Answer from the drawing. Dimensions are ordinates in mm from the lowest x, y and z of the part. A direction names the side the tool comes from. Give positions to 0.01 mm unless a question says otherwise; leave off trailing zeros. Write each loop counter-clockwise with the first axis right and the second up, starting at its lowest first coordinate (ties: lowest second). Pieces come first, ordered by that corner, then holes. Notation, with made-up numbers: (84, 60) -> (108, 60) arc R4 cw to (108, 67) -> close; hole circle Ø10 at (44.5, 56.5). An arc over 180 degrees is marked (long way). Write item = value, one per line.
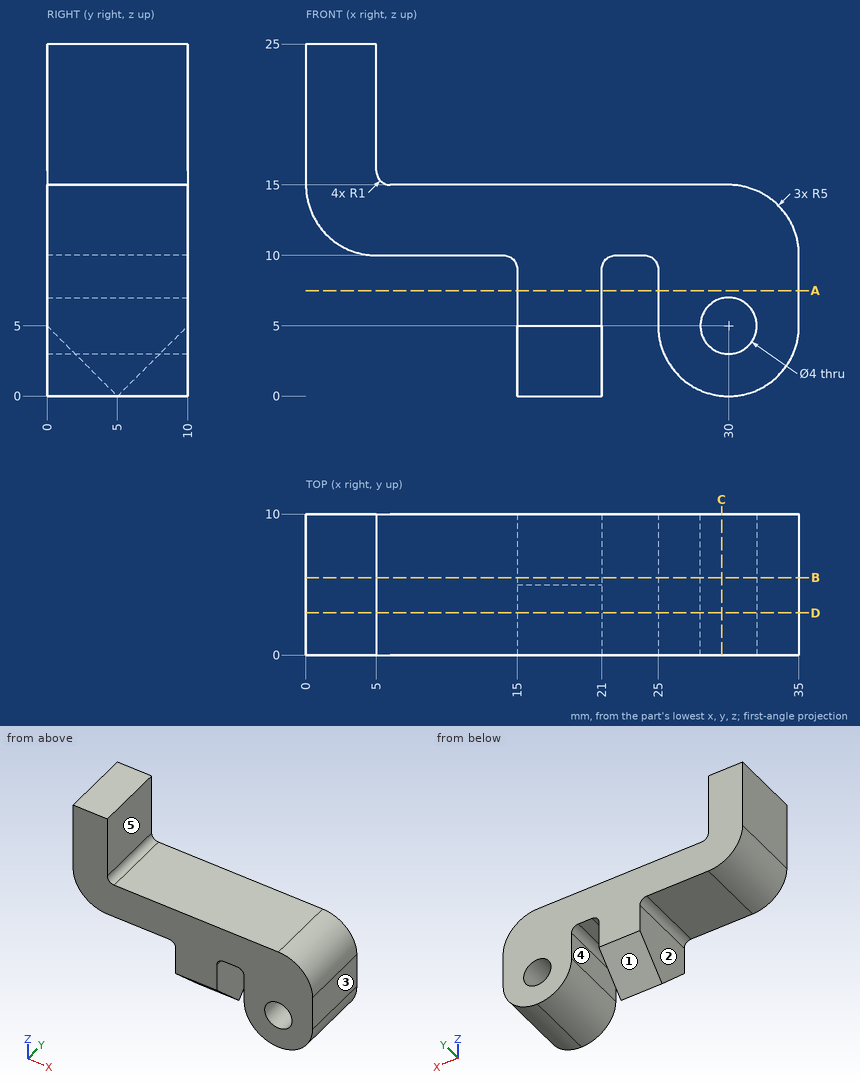
(1) The part is cut by section A-A on z = 7.5. Determine the outline of the cut face in (x, y).
Checks:
outline = (15, 0) -> (21, 0) -> (21, 10) -> (15, 10) -> close; (25, 0) -> (35, 0) -> (35, 10) -> (25, 10) -> close
(2) Consider L1, parallel to Z at x = 9, y = 6.75; L2, parallel to X at y = 8, z = 7.25; L3, parallel to X at y = 1, z = 5.75. Determine where each line is inside the solid, lowest interval first.
Checks:
L1 = 10 to 15
L2 = 15 to 21, 25 to 35
L3 = 15 to 21, 25 to 28.15, 31.85 to 35
(3) The part is cut by section B-B on y = 5.5. Determine the outline of the cut face in (x, z).
Checks:
outline = (0, 15) arc R5 ccw to (5, 10) -> (14, 10) arc R1 cw to (15, 9) -> (15, 0.5) -> (21, 0.5) -> (21, 9) arc R1 cw to (22, 10) -> (24, 10) arc R1 cw to (25, 9) -> (25, 5) arc R5 ccw to (35, 5) -> (35, 10) arc R5 ccw to (30, 15) -> (6, 15) arc R1 cw to (5, 16) -> (5, 25) -> (0, 25) -> close; hole circle Ø4 at (30, 5)
(4) A tool of negligible diameter and unlimited length cuts with its end or side. For the marked faces 1, 2, 3, 4 and 5, from which of +Z, -Z, +X, -X, +Y, -Y can it reach the whole face along a straight path? Write none if from no direction.
Checks:
face_1 = -Z, -X, +Y
face_2 = -Z, -X, +Y, -Y
face_3 = +Z, -Z, +X, +Y, -Y
face_4 = -Z, +Y, -Y
face_5 = +Z, +X, +Y, -Y
(5) The part is cut by section C-C on x = 29.5. Determine the outline of the cut face in (y, z), plus the area to 3 significant figures.
Checks:
outline = (0, 0.03) -> (10, 0.03) -> (10, 3.06) -> (0, 3.06) -> close; (0, 6.94) -> (10, 6.94) -> (10, 15) -> (0, 15) -> close
area = 111 mm²
(6) Given P1, Ø2.5, axis at y = 6.5, z = 18.5, coming from the +X side; P2, Ø1, axis at x = 22.5, y = 3, coming from the -Z side; P3, Ø2.5, axis at y = 4, z = 3, coming from the +X side; P4, Ø3.5, axis at x = 30, z = 5, coming from the +Y side, each flat-ended and moving along its own axis, determine where each tip first touches the part or whether it passes through.
Checks:
P1 = 5
P2 = 10
P3 = 34.94
P4 = through
(7) The part is cut by section D-D on y = 3. Determine the outline of the cut face in (x, z), plus the area to 3 significant figures.
Checks:
outline = (0, 15) arc R5 ccw to (5, 10) -> (14, 10) arc R1 cw to (15, 9) -> (15, 2) -> (21, 2) -> (21, 9) arc R1 cw to (22, 10) -> (24, 10) arc R1 cw to (25, 9) -> (25, 5) arc R5 ccw to (35, 5) -> (35, 10) arc R5 ccw to (30, 15) -> (6, 15) arc R1 cw to (5, 16) -> (5, 25) -> (0, 25) -> close; hole circle Ø4 at (30, 5)
area = 340 mm²
